from build123d import *

# Parameters (mm, degrees)
SKETCH1_W           = 224
SKETCH1_H           = 364
BOSS_EXTRUDE1_DEPTH = 16
SKETCH2_R           = 52.15
SKETCH2_R_2         = 87.8
CUT_EXTRUDE1_DEPTH  = 4
SKETCH3_R           = 40
SKETCH3_R_2         = 73
CUT_EXTRUDE2_DEPTH  = 17


with BuildPart() as part:
    # Sketch1 → Boss-Extrude1 (new body)
    with BuildSketch(Plane.XY):
        Rectangle(SKETCH1_W, SKETCH1_H)
    extrude(amount=BOSS_EXTRUDE1_DEPTH)

    # Sketch2 → Cut-Extrude1 (cut)
    with BuildSketch(Plane.XY.offset(16)):
        with Locations((0, 109)):
            Circle(SKETCH2_R)
        with Locations((0, -44)):
            Circle(SKETCH2_R_2)
    extrude(amount=-CUT_EXTRUDE1_DEPTH, mode=Mode.SUBTRACT)

    # Sketch3 → Cut-Extrude2 (cut, through all)
    with BuildSketch(Plane.XY.offset(16)):
        with Locations((0, 109)):
            Circle(SKETCH3_R)
        with Locations((0, -44)):
            Circle(SKETCH3_R_2)
    extrude(amount=-CUT_EXTRUDE2_DEPTH, mode=Mode.SUBTRACT)


solid = part.part
For this review, take the finished solid that the model builds, in its own axes (mm). A direction names the side the tool comes from. Round coordinates to 2 decimals unless told otherwise and drop trailing zeros. Order: outer loops, then holes, each group sorted by start corner. A loop starts at its lowest first (then second) coordinate and runs counter-clockwise, first axis right, second up. Notation, with made-up numbers: (31.25, 75) -> (39.25, 75) arc R22 cw to (39.25, 109) -> close; hole circle Ø4 at (3, -3). An arc over 180 degrees is marked (long way). Put each result on its own line as item: value.
Q1. Add section A-A on y = 109. Write out the cut boundary in (x, z).
Check result:
outline: (-112, 0) -> (-40, 0) -> (-40, 12) -> (-52.15, 12) -> (-52.15, 16) -> (-112, 16) -> close; (40, 0) -> (112, 0) -> (112, 16) -> (52.15, 16) -> (52.15, 12) -> (40, 12) -> close
Q2. Mouldability with a two-part tool opening along X and no side actions: class faces 3 (the flat face through (-112, -3, 8)), 4 (the flat face through (-2, -182, 8)), 5 (the flat face through (13, 28, 12)) as pulls with the +X half, pulls with the -X half, needs draft (parallel to the pull), parting line crosses it, or undercut.
Check result:
face 3: pulls with the -X half
face 4: needs draft
face 5: undercut
Q3. For probe 1 along Y at (x, z) = (2.5, 4.5); probe 2 along Y at (x, z) = (2, 7.25); probe 3 along Z at (x, y) = (-51, 102), list the stretches that pass through material, from the lowest coordinate up. Write a range as [from, to].
Check result:
probe 1: [-182, -116.96], [28.96, 69.08], [148.92, 182]
probe 2: [-182, -116.97], [28.97, 69.05], [148.95, 182]
probe 3: [0, 12]
Q4. Add section D-D on y = -44. Write out the cut boundary in (x, z), plus the area to 3 significant figures.
Check result:
outline: (-112, 0) -> (-73, 0) -> (-73, 12) -> (-87.8, 12) -> (-87.8, 16) -> (-112, 16) -> close; (73, 0) -> (112, 0) -> (112, 16) -> (87.8, 16) -> (87.8, 12) -> (73, 12) -> close
area: 1,130 mm2
Q5. Machinability: for faces 1 (the cylindrical face through (-15.825, -115.264, 6.084)), 2 (the cylindrical face through (-11.31, 58.09, 14.03)), which of the approach directions +Z, -Z, +X, -X, +Y, -Y give a long, thin tool a straight path to every point of the face, cutting with its end or side? Answer none if there is none.
Check result:
face 1: +Z, -Z
face 2: +Z
Q6. Add section C-C on z = 3.5. Write out the cut boundary in (x, y).
Check result:
outline: (-112, -182) -> (112, -182) -> (112, 182) -> (-112, 182) -> close; hole circle Ø146 at (0, -44); hole circle Ø80 at (0, 109)
Q7. Add section B-B on x = 0. Write out the cut boundary in (y, z), plus the area to 3 significant figures.
Check result:
outline: (-182, 0) -> (-117, 0) -> (-117, 12) -> (-131.8, 12) -> (-131.8, 16) -> (-182, 16) -> close; (29, 0) -> (69, 0) -> (69, 12) -> (56.85, 12) -> (56.85, 16) -> (43.8, 16) -> (43.8, 12) -> (29, 12) -> close; (149, 0) -> (182, 0) -> (182, 16) -> (161.15, 16) -> (161.15, 12) -> (149, 12) -> close
area: 1,990 mm2
